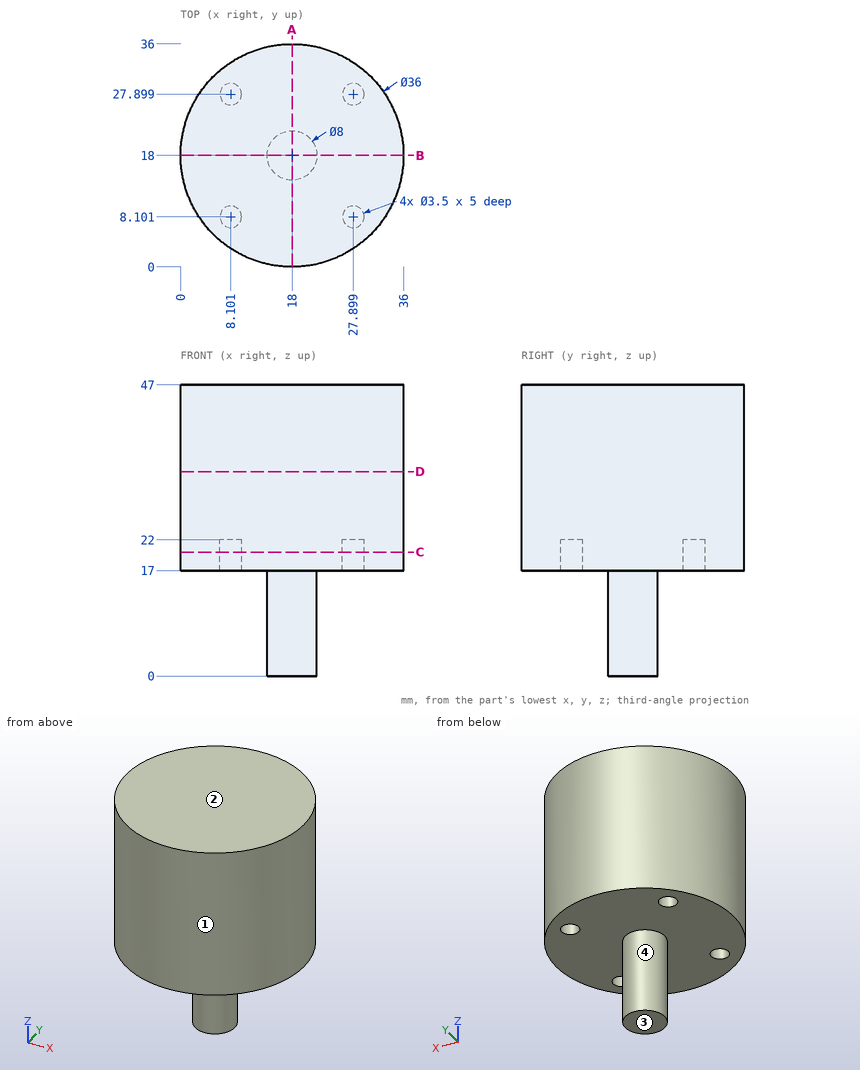
Design review of the part shown in the three views and the two pictorial views. Dimensions are in mm from the part's minimum x, y and z. A direction names the side the tool comes from. Round coordinates to 2 decimals unless told otherwise and drop trailing zeros. Loops run counter-clockwise (first coordinate to the right, second up) from the corner with the lowest first, then second, coordinate; pieces in that order, holes last. Notation, with made-up numbers: (32.5, 46.5) -> (73.5, 46.5) arc R25 ccw to (73.5, 69.5) -> close; hole circle Ø5 at (-39, -28.5). An arc over 180 degrees is marked (long way). Return JSON: item names as keys, results as strings.
(1) Add section D-D on z = 33. Write out the cut boundary in (x, y), plus the area to 3 significant figures.
Solved:
{"outline": "circle Ø36 at (18, 18)", "area": "1,020 mm2"}
(2) The part is to be moulded in two halves that separate along Y. For the marked faces 1 and 2, say which applies: released by +Y, released by -Y, zero draft, split by the parting line, or undercut.
Solved:
{"face 1": "split by the parting line", "face 2": "zero draft"}
(3) For line 1 (Y direction, x = 8.5, z = 21) (1 decimal); line 2 (Z direction, x = 11, y = 29); line 3 (X direction, y = 25.5, z = 43), list the stretches that pass through material, from the lowest coordinate up.
Solved:
{"line 1": "2.7 to 6.4, 9.8 to 26.2, 29.6 to 33.3", "line 2": "17 to 47", "line 3": "1.64 to 34.36"}
(4) For the marked faces 3 and 4, list the 3-axis set-ups (+Z, -Z, +X, -X, +Y, -Y) from which the entire face can be reached by the end or side of a thin tool; tool diameter is ignored.
Solved:
{"face 3": "-Z, +X, -X, +Y, -Y", "face 4": "-Z"}
(5) Add section A-A on x = 18. Write out the cut boundary in (y, z).
Solved:
{"outline": "(0, 17) -> (14, 17) -> (14, 0) -> (22, 0) -> (22, 17) -> (36, 17) -> (36, 47) -> (0, 47) -> close"}
(6) For pin 1 (1.5 mm diameter, centred on x = 14.5, y = 30.5, fed in from -Z); pin 2 (18 mm diameter, centred on x = 19.5, y = 24, fed in from -Z); pin 3 (6 mm diameter, centred on y = 26, z = 10.5, fed in from +X); pin 4 (2 mm diameter, centred on x = 8.1, y = 27.9, fed in from -Z), all flat-tipped, find the tip position at first contact; note any pin that passes through.
Solved:
{"pin 1": "z = 17", "pin 2": "z = 0", "pin 3": "through", "pin 4": "z = 22"}
(7) Add section C-C on z = 20. Write out the cut boundary in (x, y).
Solved:
{"outline": "circle Ø36 at (18, 18); hole circle Ø3.5 at (8.1, 8.1); hole circle Ø3.5 at (8.1, 27.9); hole circle Ø3.5 at (27.9, 8.1); hole circle Ø3.5 at (27.9, 27.9)"}
